```python
from build123d import *

# Parameters (mm, degrees)
BOSS_EXTRUDE2_DEPTH = 40
CUT_EXTRUDE1_DEPTH  = 20
SKETCH4_W           = 20
SKETCH4_H           = 20
CUT_EXTRUDE2_DEPTH  = 10


with BuildPart() as part:
    # Sketch2 → Boss-Extrude2 (new body)
    with BuildSketch(Plane(origin=(0, 0, 0), x_dir=(1, 0, 0), z_dir=(0, 1, 0))):
        Polygon((0, 0), (80, 0), (80, -60), (30, -60), (30, -20), (10, -20), (10, -10), (0, -10), align=None)
    extrude(amount=BOSS_EXTRUDE2_DEPTH)

    # Sketch3 → Cut-Extrude1 (cut)
    with BuildSketch(Plane(origin=(0, 40, 0), x_dir=(1, 0, 0), z_dir=(0, 1, 0))):
        Polygon((80, -52.352661089), (80, -60), (30, -60), (30, -20), (60, -20), (60, -50), (80, -50), align=None)
    extrude(amount=-CUT_EXTRUDE1_DEPTH, mode=Mode.SUBTRACT)

    # Sketch4 → Cut-Extrude2 (cut)
    with BuildSketch(Plane(origin=(0, 20, 0), x_dir=(1, 0, 0), z_dir=(0, 1, 0))):
        with Locations((40, -50)):
            Rectangle(SKETCH4_W, SKETCH4_H)
    extrude(amount=-CUT_EXTRUDE2_DEPTH, mode=Mode.SUBTRACT)


solid = part.part
```
Check sheet for the modelled part. Datum: model origin and axes. Units: mm. A direction names the side the tool comes from. Coordinates: 2 decimals unless noted, no trailing zeros. Order: outer loops, then holes, each group sorted by start corner. A loop starts at its lowest first (then second) coordinate and runs counter-clockwise, first axis right, second up. Notation, with made-up numbers: (67, -27.5) -> (108, -27.5) arc R18 cw to (108, -12.5) -> close; hole circle Ø9 at (67.25, 7). An arc over 180 degrees is marked (long way). Write each question's results on one line, items separated by ' | '. Start each with the question number.
1) Material ranges on line 1 along X through (y, z) = (15, 48.5); line 2 along Z through (x, y) = (14, 23); line 3 along Z through (x, y) = (64, 35), recorded low to high.
2) Depth check by flat-ended pin: pin 1 (22 mm diameter, centred on x = 43, z = 50.5, fed in from +Y); pin 2 (4 mm diameter, centred on y = 9, z = 13.5, fed in from -X); pin 3 (2 mm diameter, centred on y = 36, z = 21.5, fed in from -X). Enter the tip coordinate at first touch or a pass-through.
3) Set-up check for faces 1 (the face through (40, 15, 40)), 2 (the face through (70, 30, 50)), 3 (the face through (5, 20, 10)): record each of +Z, -Z, +X, -X, +Y, -Y from which the full face is reachable in a straight line by a thin tool's end or side.
4) Section check D-D (y = 18). Enter the section's corners in (x, z), and give its area (3 significant figures).
5) Section check C-C (z = 23). Enter the section's corners in (x, y).
6) Section check B-B (x = 46). Enter the section's corners in (y, z), and give its area (3 significant figures).
7) Section check A-A (y = 4.5). Enter the section's corners in (x, z), and give its area (3 significant figures).
Checked values:
1) line 1: 50 to 80 | line 2: 0 to 20 | line 3: 0 to 50
2) pin 1: y = 20 | pin 2: x = 10 | pin 3: x = 60
3) face 1: +Z, -X, +Y | face 2: +Z, +X, -X, +Y | face 3: +Z, -X, +Y, -Y
4) outline: (0, 0) -> (80, 0) -> (80, 60) -> (50, 60) -> (50, 40) -> (30, 40) -> (30, 20) -> (10, 20) -> (10, 10) -> (0, 10) -> close | area: 3,100 mm²
5) outline: (30, 0) -> (80, 0) -> (80, 40) -> (60, 40) -> (60, 20) -> (30, 20) -> close
6) outline: (0, 0) -> (40, 0) -> (40, 20) -> (20, 20) -> (20, 40) -> (10, 40) -> (10, 60) -> (0, 60) -> close | area: 1,400 mm²
7) outline: (0, 0) -> (80, 0) -> (80, 60) -> (30, 60) -> (30, 20) -> (10, 20) -> (10, 10) -> (0, 10) -> close | area: 3,500 mm²
